Input: part model. Units: mm. Frame: model coordinates. Face numbers are marked on the shaded views. Round coordinates to 2 decimals unless told otherwise and drop trailing zeros. Loops run counter-clockwise (first coordinate to the right, second up) from the corner with the lowest first, then second, coordinate; pieces in that order, holes last. Notation, with made-up numbers: (45, 35.25) - (57, 35.25) arc R19 ccw to (57, 39.25) - close; hole circle Ø9 at (82, -3). An arc over 180 degrees is marked (long way). One line per question, with ' | ' between items. Start each with the question number.
from build123d import *

# Parameters (mm, degrees)
SKETCH3_W           = 3.6
SKETCH3_H           = 2.8
SKETCH3_RX          = 1
SKETCH3_RY          = 0.75
BOSS_EXTRUDE1_DEPTH = 0.25


with BuildPart() as part:
    # Sketch2 → Revolve1 (revolve)
    with BuildSketch(Plane(origin=(0, 0, 0), x_dir=(1, 0, 0), z_dir=(0, 1, 0))):
        with BuildLine():
            Line((0, 8.75), (-2.5, 8.75))
            Line((-2.5, 8.75), (-5.5, 6.9))
            Line((-5.5, 6.9), (-5.5, 5.9))
            add(Edge.make_bspline(
                [(-5.5, 5.9), (-6.436492627, 5.9), (-8.1, 5.494365828), (-8.1, 3)],
                knots=[0, 0, 0, 0, 1, 1, 1, 1], degree=3))
            Line((-8.1, 3), (-8.1, 0))
            Line((-8.1, 0), (0, 0))
            Line((0, 0), (9.9, 0))
            Line((9.9, 0), (9.9, 4.5))
            Line((9.9, 4.5), (9.4, 4.5))
            Line((9.4, 4.5), (8.9, 5))
            Line((8.9, 5), (7.9, 5))
            Line((7.9, 5), (6.9, 6))
            Line((6.9, 6), (0, 6))
            Line((0, 6), (0, 8.75))
        make_face()
    revolve(axis=Axis((0, 0, 0), (-1, 0, 0)))

    # Sketch3 → Boss-Extrude1 (add, symmetric)
    with BuildSketch(Plane.XY.offset(2.3)):
        with Locations((11.7, 0)):
            Rectangle(SKETCH3_W, SKETCH3_H)
        with Locations((11.8, 0)):
            Ellipse(SKETCH3_RX, SKETCH3_RY, mode=Mode.SUBTRACT)
    boss_extrude1 = extrude(amount=BOSS_EXTRUDE1_DEPTH, both=True)

    # Mirror1: Boss-Extrude1 across plane
    add(boss_extrude1.mirror(Plane.XY))


solid = part.part
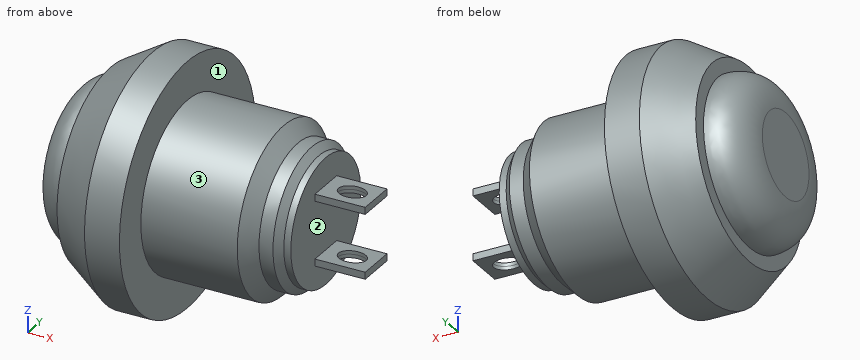
(1) Line query: line 1 along Z through (x, y) = (10.25, -1.25); line 2 along X through (y, z) = (0.5, -0.75); line 3 along Z through (x, y) = (0.5, 0.25). Output: solid intervals per line, ascending. Write a range as from..to.
(2) Section D-D, the plane x = 5.75. Output: boundary loops of the cut face in (y, z).
(3) Section A-A, the plane y = 0. Give the number of separate pieces and of enclosed holes in the cut face, plus the area to 3 significant figures.
(4) Section B-B, the plane x = 8.5. Output: boundary loops of the cut face in (y, z), plus the area to 3 significant figures.
(5) Pin query (flat end, axial travel): P1, Ø4, axis at x = 8, y = 3, coming from the +Z side; P2, Ø2, axis at y = 2, z = 1, coming from the +X side; P3, Ø6, axis at x = 2.5, y = -2.5, coming from the +Z side. Return the tip coordinate at first contact, or that it passes through.
(6) Pull-direction query (Z, two-part tool) for the marked faces 1, 2 and 3; classes: released by +Z, released by -Z, zero draft, split by the parting line, or undercut.
Derived:
1) line 1: z = -2.55..-2.05, 2.05..2.55 | line 2: x = -8.1..9.9 | line 3: z = -5.99..5.99
2) outline: circle Ø12 at (0, 0)
3) separate pieces: 3 | enclosed holes: 0 | area: 233 mm²
4) outline: circle Ø10 at (0, 0) | area: 78.5 mm²
5) P1: stops at z = 5.85 | P2: stops at x = 9.9 | P3: stops at z = 8.71
6) face 1: zero draft | face 2: undercut | face 3: split by the parting line
